Could you check a few things on this model? Use its own coordinates, in mm. A direction names the side the tool comes from. Give positions to 0.01 mm unless a question says otherwise; leave off trailing zeros. Loops run counter-clockwise (first coordinate to the right, second up) from the corner with the lowest first, then second, coordinate; pieces in that order, holes last. Notation, with made-up numbers: (89.5, 33) - (102.5, 33) arc R20 cw to (102.5, 60) - close; hole circle Ø6 at (-23.75, -10.5). An arc over 180 degrees is marked (long way). One line per item, written item: value. Start each with the question number.
Q1. If we mould it in two halves opening along X, with no side actions, what happens to faces 3 (the face through (4.53, -4.56, 0.43)), 4 (the face through (0, -4, -22.75)), 5 (the face through (16.713, 17.255, -14.564)), 6 (the face through (-24.5, -4, -7))? For each: released by +X, released by -X, zero draft, split by the parting line, or undercut.
Q2. I'm going to push flat-ended pins straight in: P1, Ø6, axis at x = -6, y = 3.5, coming from the +Z side; P2, Ø23, axis at x = -11, z = -11, coming from the +Y side; P3, Ø1.5, axis at x = -17.5, y = 6.5, coming from the -Z side. Where does each tip first touch, or does it pass through?
Q3. If I drill on line 1 (Z direction, x = 0, y = -2.75); line 2 (Y direction, x = 1.5, z = -12.5); line 3 (X direction, y = -7, z = 3), over which ranges is the centre line in solid material (lowest first)? Write a range as from..to.
Q4. I want a section at C-C (z = -15.3). Please give me the cut outline in (x, y), then the cut area to 3 significant figures.
Q5. I want a section at D-D (x = 18). Please give me the cut outline in (y, z), then the cut area to 3 significant figures.
Q6. For faces 1 (the face through (-6, -9, 0)), 2 (the face through (-16.602, 17.255, -15.192)), which set-ups out of +Z, -Z, +X, -X, +Y, -Y let a thin tool reach every point of the face, with its end or its side?
Q7. I want a section at B-B (y = 5.5). Please give me the cut outline in (x, z).
Q8. I want a section at A-A (x = 0). Please give me the cut outline in (y, z).
```python
from build123d import *

# Parameters (mm, degrees)
F1_DEPTH = 9
F2_R     = 4.75
F3_DEPTH = 25
F4_R     = 2.45
F5_DEPTH = 35


with BuildPart() as f1:
    # F0 (on Front) → F1 (new body)
    with BuildSketch(Plane.XZ):
        with BuildLine():
            Line((-24.5, -22.75), (24.5, -22.75))
            Line((24.5, -22.75), (24.5, 7.75))
            ThreePointArc((24.5, 7.75), (20.106602, 18.356602), (9.5, 22.75))
            Line((9.5, 22.75), (-9.5, 22.75))
            ThreePointArc((-9.5, 22.75), (-20.106602, 18.356602), (-24.5, 7.75))
            Line((-24.5, 7.75), (-24.5, -22.75))
        make_face()
    extrude(amount=F1_DEPTH)

    # F2 (on face) → F3 (cut)
    with BuildSketch(Plane.XZ.offset(9)):
        with Locations((0, -1)):
            Circle(F2_R)
    extrude(amount=-F3_DEPTH, mode=Mode.SUBTRACT)

    # F4 (on face) → F5 (join)
    with BuildSketch(Plane(origin=(0, 0, 0), x_dir=(-1, 0, 0), z_dir=(0, 1, 0))):
        with Locations((-19.05, -15.3)):
            Circle(F4_R)
        with Locations((19.05, -15.3)):
            Circle(F4_R)
    extrude(amount=F5_DEPTH)


solid = f1.part
```
Worked answers:
1. face 3: undercut
1. face 4: zero draft
1. face 5: undercut
1. face 6: released by -X
2. P1: passes through
2. P2: stops at y = 35
2. P3: stops at z = -17.62
3. line 1: z = -22.75..-5.75, 3.75..22.75
3. line 2: y = -9..0
3. line 3: x = -24.5..-2.56, 2.56..24.5
4. outline: (-24.5, -9) - (24.5, -9) - (24.5, 0) - (21.5, 0) - (21.5, 35) - (16.6, 35) - (16.6, 0) - (-16.6, 0) - (-16.6, 35) - (-21.5, 35) - (-21.5, 0) - (-24.5, 0) - close
4. area: 784 mm²
5. outline: (-9, -22.75) - (0, -22.75) - (0, -17.51) - (35, -17.51) - (35, -13.09) - (0, -13.09) - (0, 20.11) - (-9, 20.11) - close
5. area: 541 mm²
6. face 1: +Z, -Z, +X, -X, -Y
6. face 2: +Y
7. outline: circle Ø4.9 at (-19.05, -15.3); circle Ø4.9 at (19.05, -15.3)
8. outline: (-9, -22.75) - (0, -22.75) - (0, -5.75) - (-9, -5.75) - close; (-9, 3.75) - (0, 3.75) - (0, 22.75) - (-9, 22.75) - close
